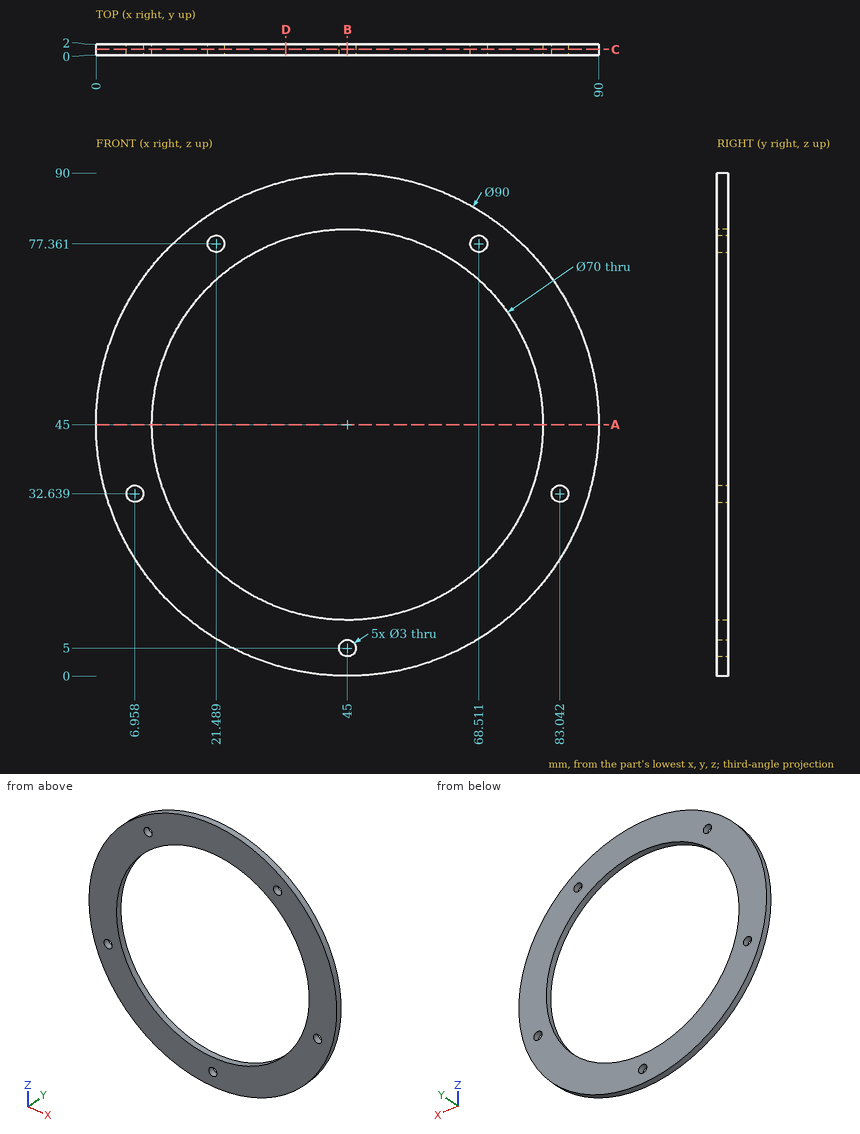
Source: three-view drawing plus pictorial views. Frame: mm from the lowest corner of the part. Coordinates: 2 decimals unless noted, no trailing zeros. Order: outer loops, then holes, each group sorted by start corner. A loop starts at its lowest first (then second) coordinate and runs counter-clockwise, first axis right, second up. Notation, with made-up numbers: (25.25, 55) -> (49.25, 55) arc R18 ccw to (49.25, 81) -> close; hole circle Ø2 at (75.25, 71.25). An arc over 180 degrees is marked (long way). Write item = value, one per line.
(1) Cut plane D-D on x = 34. Return loops of the section in (y, z) (1 decimal).
Solved:
outline = (0, 1.4) -> (2, 1.4) -> (2, 11.8) -> (0, 11.8) -> close; (0, 78.2) -> (2, 78.2) -> (2, 88.6) -> (0, 88.6) -> close
(2) Cut plane A-A on z = 45. Return loops of the section in (x, y).
Solved:
outline = (0, 0) -> (10, 0) -> (10, 2) -> (0, 2) -> close; (80, 0) -> (90, 0) -> (90, 2) -> (80, 2) -> close
(3) Line query: line 1 (Z direction, x = 45, y = 1.1); line 2 (X direction, y = 0.55, z = 46) (1 decimal); line 3 (Z direction, x = 46, y = 1.9) (1 decimal). Output: solid intervals per line, ascending.
Solved:
line_1 = 0 to 3.5, 6.5 to 10, 80 to 90
line_2 = 0 to 10, 80 to 90
line_3 = 0 to 3.9, 6.1 to 10, 80 to 90
(4) Cut plane C-C on y = 1.05. Return loops of the section in (x, z), plus the area to 3 significant figures.
Solved:
outline = circle Ø90 at (45, 45); hole circle Ø3 at (6.96, 32.64); hole circle Ø70 at (45, 45); hole circle Ø3 at (21.49, 77.36); hole circle Ø3 at (45, 5); hole circle Ø3 at (68.51, 77.36); hole circle Ø3 at (83.04, 32.64)
area = 2,480 mm²
(5) Cut plane B-B on x = 45. Return loops of the section in (y, z).
Solved:
outline = (0, 0) -> (2, 0) -> (2, 3.5) -> (0, 3.5) -> close; (0, 6.5) -> (2, 6.5) -> (2, 10) -> (0, 10) -> close; (0, 80) -> (2, 80) -> (2, 90) -> (0, 90) -> close
(6) Pin query (flat end, axial travel): pin 1 Ø8 at (x, z) = (65.5, 66) entering from -Y (3 decimals). Return the tip coordinate at first contact, or that it passes through.
Solved:
pin_1 = through
